Could you check a few things on this drawing? It's one solid part, dimensions in mm from its lowest x, y, z. Round coordinates to 2 decimals unless told otherwise and drop trailing zeros. Loops run counter-clockwise (first coordinate to the right, second up) from the corner with the lowest first, then second, coordinate; pieces in that order, holes last. Notation, with made-up numbers: M 65.25,1 L 86.25,1 A24 ccw 86.25,25 Z; hole C -7,-25.5 d11. An arc over 180 degrees is marked long. Return JSON: item names as keys, results as strings.
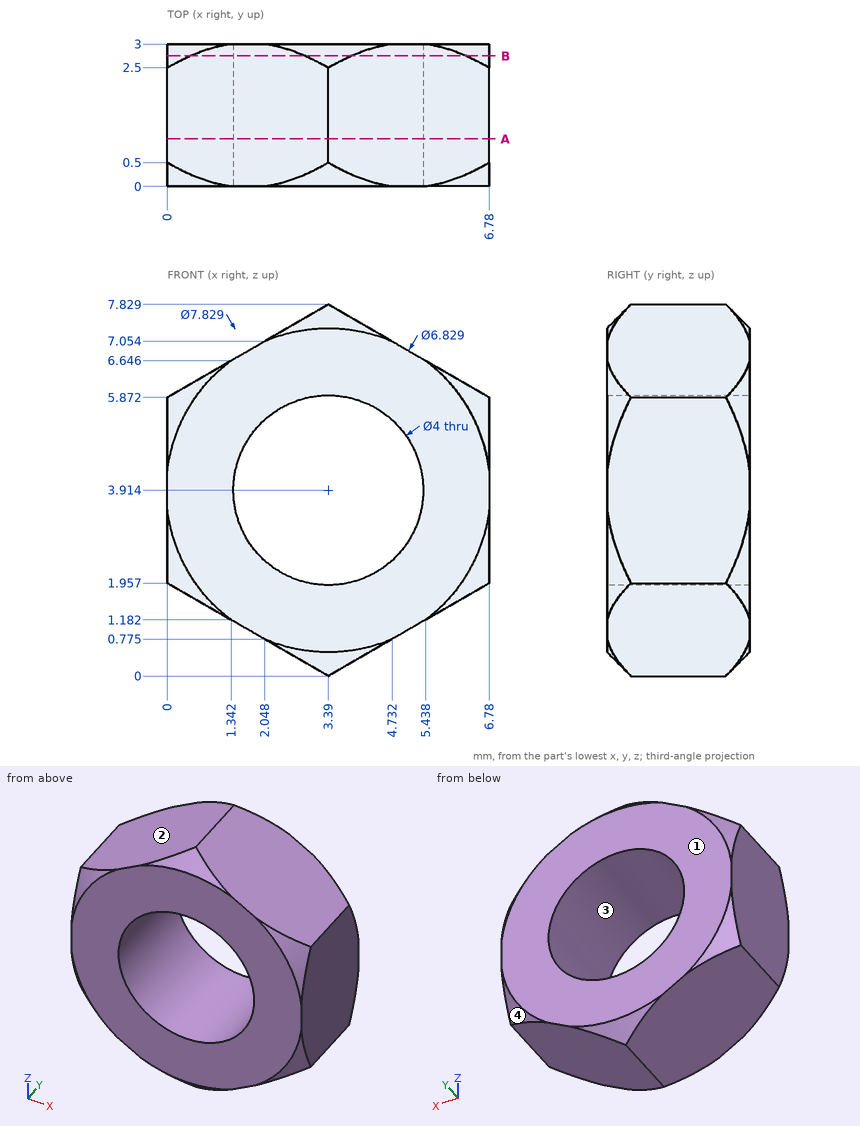
Q1. Suppose I cut it at B-B, the plane y = 2.75. Please give me the cut outline in (x, z) (1 decimal).
Results:
{"outline": "M 0,2.5 A3.7 ccw 0.5,1.7 L 2.9,0.3 A3.7 ccw 3.9,0.3 L 6.3,1.7 A3.7 ccw 6.8,2.5 L 6.8,5.3 A3.7 ccw 6.3,6.2 L 3.9,7.5 A3.7 ccw 2.9,7.5 L 0.5,6.2 A3.7 ccw 0,5.3 Z; hole C 3.4,3.9 d4"}
Q2. Suppose I cut it at A-A, the plane y = 1. Please give me the cut outline in (x, z) (1 decimal).
Results:
{"outline": "M 0,2 L 3.4,0 L 6.8,2 L 6.8,5.9 L 3.4,7.8 L 0,5.9 Z; hole C 3.4,3.9 d4"}
Q3. If I drill on line 1 along X through (y, z) = (0.6, 4); line 2 along Z through (x, y) = (4, 1.55) (1 decimal); line 3 along X through (y, z) = (1.4, 5.75) (1 decimal), over which ranges is the centre line in solid material (lowest first)?
Results:
{"line 1": "x = 0 to 1.39, 5.39 to 6.78", "line 2": "z = 0.4 to 2, 5.8 to 7.5", "line 3": "x = 0 to 2.6, 4.2 to 6.8"}
Q4. Thinking about a two-plate mould opening in Z: for the marked faces 1, 2, 3 and 4, which applies, pulls with the +Z half, pulls with the -Z half, needs draft (parallel to the pull), parting line crosses it, or undercut?
Results:
{"face 1": "needs draft", "face 2": "pulls with the +Z half", "face 3": "undercut", "face 4": "pulls with the -Z half"}
